The listing builds one solid part. Answer for the finished solid, in the listing's coordinates (mm). Give positions to 0.01 mm unless a question says otherwise; leave off trailing zeros. Loops run counter-clockwise (first coordinate to the right, second up) from the corner with the lowest first, then second, coordinate; pieces in that order, holes last. Notation, with made-up numbers: M 44,-13.75 L 71,-13.75 A21 cw 71,9.25 Z; hole C 56,61 d4. An arc over 180 degrees is marked long. Return JSON: item names as keys, results as strings.
from build123d import *

# Parameters (mm, degrees)
SKETCH2_W           = 45
SKETCH2_H           = 20
BOSS_EXTRUDE1_DEPTH = 28
SKETCH3_R           = 1.5
CUT_EXTRUDE1_DEPTH  = 28


with BuildPart() as part:
    # Sketch2 → Boss-Extrude1 (new body)
    with BuildSketch(Plane.XY):
        with Locations((22.5, 10)):
            Rectangle(SKETCH2_W, SKETCH2_H)
    extrude(amount=-BOSS_EXTRUDE1_DEPTH)

    # Sketch3 → Cut-Extrude1 (cut)
    with BuildSketch(Plane.XY):
        with Locations((22.5, 10.010662988)):
            Circle(SKETCH3_R)
        with Locations((19, 17.000059599)):
            Circle(SKETCH3_R)
        with Locations((19, 2.999940401)):
            Circle(SKETCH3_R)
        with Locations((26, 2.999940401)):
            Circle(SKETCH3_R)
        with Locations((26, 17.000059599)):
            Circle(SKETCH3_R)
    extrude(amount=-CUT_EXTRUDE1_DEPTH, mode=Mode.SUBTRACT)


solid = part.part
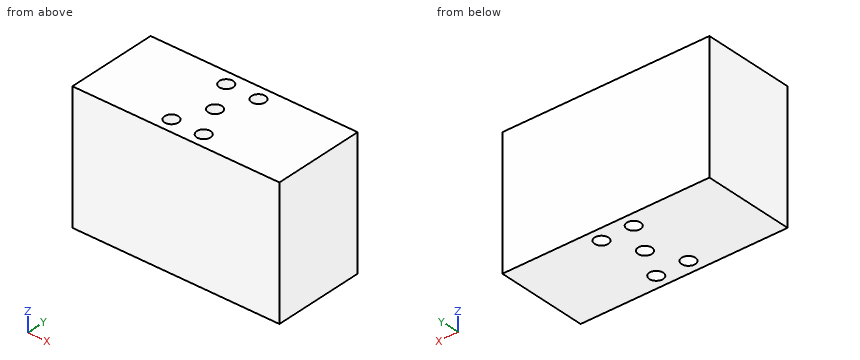
(1) Given pin 1 (4 mm diameter, centred on x = 5.5, z = -12.5, fed in from -Y); pin 2 (1.8 mm diameter, centred on x = 26, y = 3, fed in from +Z), each flat-ended and moving along its own axis, determine where each tip first touches the part or whether it passes through.
Values follow:
{"pin 1": "y = 0", "pin 2": "through"}
(2) The part is cut by section B-B (z = -23.75). Determine the outline of the cut face in (x, y).
Values follow:
{"outline": "M 0,0 L 45,0 L 45,20 L 0,20 Z; hole C 19,3 d3; hole C 19,17 d3; hole C 22.5,10.01 d3; hole C 26,3 d3; hole C 26,17 d3"}
(3) The part is cut by section A-A (x = 22.5). Determine the outline of the cut face in (y, z).
Values follow:
{"outline": "M 0,-28 L 8.51,-28 L 8.51,0 L 0,0 Z; M 11.51,-28 L 20,-28 L 20,0 L 11.51,0 Z"}
(4) The part is cut by section C-C (y = 3.75). Determine the outline of the cut face in (x, z), and give its area (3 significant figures).
Values follow:
{"outline": "M 0,-28 L 17.7,-28 L 17.7,0 L 0,0 Z; M 20.3,-28 L 24.7,-28 L 24.7,0 L 20.3,0 Z; M 27.3,-28 L 45,-28 L 45,0 L 27.3,0 Z", "area": "1,110 mm²"}
(5) Straight lines are drawn through the part: line 1 along Y through (x, z) = (26, -16.5); line 2 along Y through (x, z) = (22.5, -18); line 3 along X through (y, z) = (17.25, -15.25). For each, find the intervals that lie inside material, in ascending order.
Values follow:
{"line 1": "0 to 1.5, 4.5 to 15.5, 18.5 to 20", "line 2": "0 to 8.51, 11.51 to 20", "line 3": "0 to 17.52, 20.48 to 24.52, 27.48 to 45"}
